Part model, mm, in its own coordinate system. A direction names the side the tool comes from. Round coordinates to 2 decimals unless told otherwise and drop trailing zeros. Loops run counter-clockwise (first coordinate to the right, second up) from the corner with the lowest first, then second, coordinate; pieces in that order, holes last. Notation, with made-up numbers: M 72.5,59 L 104.5,59 A17 cw 104.5,65 Z; hole C 81,16.5 d8. An arc over 180 degrees is marked long. Write each question's results on one line, items separated by ' | '.
Solid Edge part; units mm, degrees
sketch "Sketch1" plane through (0, 0, 0) normal (0, 0, 1) x (1, 0, 0)
  circle A0 centre (0, 0) radius 27.5
extrude "Protrusion1" add sketch "Sketch1" along normal blind 4.5
sketch "Sketch2" plane through (0, 0, 4.5) normal (0, 0, 1) x (0, 1, 0)
  circle A0 centre (0, 0) radius 24.3
  circle A1 centre (0, 0) radius 26.3
extrude "ExtrudedProtrusion_2" add sketch "Sketch2" along normal blind 15
sketch "Sketch3" plane through (0, 0, 4.5) normal (0, 0, 1) x (0, 1, 0)
  circle A0 centre (0, 0) radius 24.3
extrude "ExtrudedCutout_1" cut sketch "Sketch3" against normal blind 1.5
chamfer "Letörés_1" distance 1 angle 45 1 edges at (0, -26.3, 19.5)
chamfer "Letörés_2" distance 0.5 angle 45 2 edges at (-27.5, 0, 4.5) (-27.5, 0, 0)
sketch "Sketch4" plane through (0, 0, 3) normal (0, 0, 1) x (0, 1, 0)
  circle A0 centre (0, -8.5) radius 1.6
  circle A1 centre (-8.5, 0) radius 1.6
  circle A2 centre (8.5, 0) radius 1.6
  circle A3 centre (0, 8.5) radius 1.6
extrude "ExtrudedCutout_2" cut sketch "Sketch4" against normal blind 7
chamfer "Letörés_3" distance 3 angle 45 1 edges at (0, -24.3, 3)
chamfer "Letörés_4" distance 0.5 angle 45 8 edges at (-6.9, 0, 0) (-8.5, -1.6, 3) (1.6, 8.5, 0) (0, 6.9, 3) (1.6, -8.5, 0) (0, -10.1, 3) (10.1, 0, 0) (8.5, -1.6, 3)
Item 1: Band-saw the part on A-A on x = 0. Count the separate pieces of the cut face and the enclosed holes in it, and give its area (3 significant figures).
Filled sheet:
separate pieces: 3 | enclosed holes: 0 | area: 222 mm^2
Item 2: Band-saw the part on B-B on z = 7. Give the cut face in (x, y).
Filled sheet:
outline: C 0,0 d52.6; hole C 0,0 d48.6
Item 3: Drop flat-ended pins along their axis: P1, Ø8, axis at x = -8, z = 4, coming from the -Y side; P2, Ø5, axis at x = 8.5, y = 0, coming from the +Z side; P3, Ø5, axis at y = -2.5, z = 17, coming from the +X side; P4, Ø1.9, axis at x = -8.5, y = 0, coming from the +Z side. Give the stop position or say it passes through.
Filled sheet:
P1: y = -27.21 | P2: z = 3 | P3: x = 26.3 | P4: through
Item 4: Wall check: L1, parallel to X at y = 0, z = 14; L2, parallel to X at y = 1, z = 2.25. Give the ranges that are in metal, low to high.
Filled sheet:
L1: -26.3 to -24.3, 24.3 to 26.3 | L2: -27.48 to -9.75, -7.25 to 7.25, 9.75 to 27.48
Item 5: Two-plate mould, pull along Y, no slides. Class faces 1 (the cylindrical face through (-0.07, -10.1, 1.51)), 2 (the cylindrical face through (-5.961, 26.846, 2.226)), 3 (the flat face through (0, 0, 0)), 4 (the cylindrical face through (-23.72, -5.27, 12.66)): +Y half, -Y half, draft (parallel to the pull), parting line (faces both ways), or undercut.
Filled sheet:
face 1: undercut | face 2: parting line | face 3: draft | face 4: undercut
Item 6: Which spindle directions (+Z, -Z, +X, -X, +Y, -Y) get a long thin tool onto all of the face, cutting with end or side? Do faces 5 (the cylindrical face through (-6.94, -0.35, 1.51)), 6 (the cylindrical face through (1.156, -26.275, 11.402)). Say none if no direction does.
Filled sheet:
face 5: +Z, -Z | face 6: +Z
